Could you check a few things on this model? Use its own coordinates, in mm. Face numbers are marked on the shaded views. Round coordinates to 2 decimals unless told otherwise and drop trailing zeros. Loops run counter-clockwise (first coordinate to the right, second up) from the corner with the lowest first, then second, coordinate; pieces in that order, holes last.
from build123d import *

# Parameters (mm, degrees)
SKETCH097_W     = 172
SKETCH097_H     = 95
PAD059_DEPTH    = 4.5
SKETCH098_W     = 6
SKETCH098_H     = 19
POCKET036_DEPTH = 3
SKETCH099_W     = 6.3
SKETCH099_H     = 11
SKETCH099_W_2   = 6
POCKET037_DEPTH = 5
PAD060_DEPTH    = 16
POCKET038_DEPTH = 5
POCKET039_DEPTH = 9
SKETCH103_R     = 1.15
POCKET040_DEPTH = 5
SKETCH104_R     = 3.3
POCKET041_DEPTH = 3


with BuildPart() as part:
    # Sketch097 → Pad059 (new body)
    with BuildSketch(Plane.XZ):
        Rectangle(SKETCH097_W, SKETCH097_H)
    extrude(amount=PAD059_DEPTH)

    # Sketch098 (on Face6 of Pad059) → Pocket036 (cut)
    with BuildSketch(Plane.XZ.offset(4.5)):
        Polygon((64.5, 3), (69.5, 3), (69.5, 28.5), (75.5, 28.5), (75.5, 47.5), (56.5, 47.5), (56.5, 37.5), (64.5, 37.5), align=None)
        with Locations((39, 38)):
            Rectangle(SKETCH098_W, SKETCH098_H)
        Polygon((-64.5, 3), (-69.5, 3), (-69.5, 28.5), (-75.5, 28.5), (-75.5, 47.5), (-56.5, 47.5), (-56.5, 37.5), (-64.5, 37.5), align=None)
    extrude(amount=-POCKET036_DEPTH, mode=Mode.SUBTRACT)

    # Sketch099 (on Face26 of Pocket036) → Pocket037 (cut)
    with BuildSketch(Plane.XZ.offset(1.5)):
        with Locations((72.35, 42)):
            Rectangle(SKETCH099_W, SKETCH099_H)
        with Locations((39, 42)):
            Rectangle(SKETCH099_W_2, SKETCH099_H)
        with Locations((-72.35, 42)):
            Rectangle(SKETCH099_W, SKETCH099_H)
    extrude(amount=-POCKET037_DEPTH, mode=Mode.SUBTRACT)

    # Sketch100 (on Face5 of Pocket037) → Pad060 (join)
    with BuildSketch(Plane.XZ.offset(4.5)):
        Polygon((-69.5, 28.5), (-71.5, 28.5), (-71.5, 1), (-62.5, 1), (-62.5, 37.5), (-64.5, 37.5), (-64.5, 3), (-69.5, 3), align=None)
        Polygon((64.5, 37.5), (64.5, 3), (69.5, 3), (69.5, 28.5), (71.5, 28.5), (71.5, 1), (62.5, 1), (62.5, 37.5), align=None)
    extrude(amount=PAD060_DEPTH)

    # Sketch101 (on Face27 of Pad060) → Pocket038 (cut)
    with BuildSketch(Plane(origin=(-71.5, 0, 0), x_dir=(0, 0, -1), z_dir=(-1, 0, 0))):
        with BuildLine():
            ThreePointArc((-28.5, 4.5), (-18.161779, 10.994502), (-10.5, 20.5))
            Line((-28.5, 20.5), (-10.5, 20.5))
            Line((-28.5, 4.5), (-28.5, 20.5))
        make_face()
    extrude(amount=-POCKET038_DEPTH, mode=Mode.SUBTRACT)

    # Sketch102 (on Face22 of Pocket038) → Pocket039 (cut)
    with BuildSketch(Plane(origin=(62.5, 0, 0), x_dir=(0, 0, -1), z_dir=(-1, 0, 0))):
        with BuildLine():
            Line((-37.5, 20.5), (-10.5, 20.5))
            ThreePointArc((-28.5, 4.5), (-18.161779, 10.994501), (-10.5, 20.5))
            Line((-37.5, 4.5), (-28.5, 4.5))
            Line((-37.5, 20.5), (-37.5, 4.5))
        make_face()
    extrude(amount=-POCKET039_DEPTH, mode=Mode.SUBTRACT)

    # Sketch103 (on Face4 of Pocket039) → Pocket040 (cut)
    with BuildSketch(Plane(origin=(0, 0, 0), x_dir=(1, 0, 0), z_dir=(0, 1, 0))):
        with Locations((-83, 43.5)):
            Circle(SKETCH103_R)
        with Locations((83, 43.5)):
            Circle(SKETCH103_R)
        with Locations((83, -43.5)):
            Circle(SKETCH103_R)
        with Locations((-83, -43.5)):
            Circle(SKETCH103_R)
    extrude(amount=-POCKET040_DEPTH, mode=Mode.SUBTRACT)

    # Sketch104 (on Face4 of Pocket040) → Pocket041 (cut)
    with BuildSketch(Plane(origin=(0, 0, 0), x_dir=(1, 0, 0), z_dir=(0, 1, 0))):
        with Locations((83, 43.5)):
            Circle(SKETCH104_R)
        with Locations((83, -43.5)):
            Circle(SKETCH104_R)
        with Locations((-83, -43.5)):
            Circle(SKETCH104_R)
        with Locations((-83, 43.5)):
            Circle(SKETCH104_R)
    extrude(amount=-POCKET041_DEPTH, mode=Mode.SUBTRACT)


with BuildPart() as part_1:
    # Body021 placement: moved
    add(part.part.moved(Location((0, -4, -56))))


solid = part_1.part
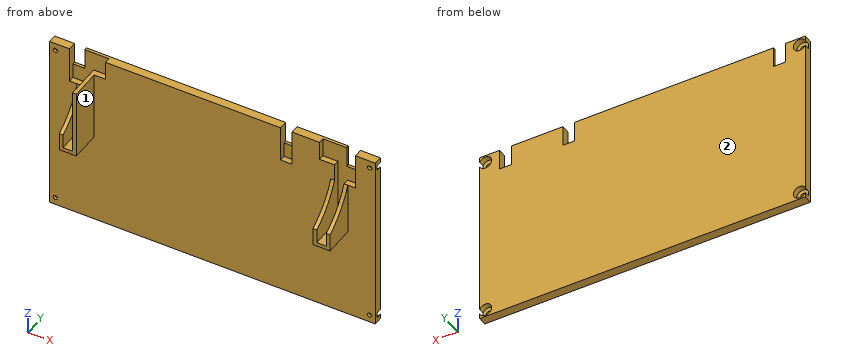
Item 1: If we section it at A-A, the plane y = -16.5: Please give me the cut outline in (x, z).
Results list:
outline: (-71.5, -55) - (-62.5, -55) - (-62.5, -18.5) - (-64.5, -18.5) - (-64.5, -53) - (-69.5, -53) - (-69.5, -39.43) - (-71.5, -39.43) - close; (62.5, -55) - (71.5, -55) - (71.5, -39.43) - (69.5, -39.43) - (69.5, -53) - (64.5, -53) - (64.5, -39.43) - (62.5, -39.43) - close
Item 2: If I drill on line 1 along X through (y, z) = (-19.75, -48); line 2 along Z through (x, y) = (-83, -7.5); line 3 along X through (y, z) = (-5.7, -12.5), over which ranges is the centre line in solid material (lowest first)?
Results list:
line 1: x = -71.5 to -69.5, -64.5 to -62.5, 62.5 to 64.5, 69.5 to 71.5
line 2: z = -103.5 to -100.65, -98.35 to -13.65, -11.35 to -8.5
line 3: x = -79.7 to -75.5, -56.5 to 36, 42 to 56.5, 75.5 to 79.7
Item 3: We'd pull the mould along X, two halves only. Please class the marked faces 1 and 2: released by +X, released by -X, zero draft, split by the parting line, or undercut.
Results list:
face 1: undercut
face 2: zero draft
Item 4: If we section it at B-B, the plane z = -50: Please give me the cut outline in (x, y).
Results list:
outline: (-86, -8.5) - (-71.5, -8.5) - (-71.5, -24.5) - (-69.5, -24.5) - (-69.5, -5.5) - (-64.5, -5.5) - (-64.5, -24.5) - (-62.5, -24.5) - (-62.5, -8.5) - (62.5, -8.5) - (62.5, -24.5) - (64.5, -24.5) - (64.5, -5.5) - (69.5, -5.5) - (69.5, -24.5) - (71.5, -24.5) - (71.5, -8.5) - (86, -8.5) - (86, -4) - (-86, -4) - close
Item 5: Will these pins go through, and if not, where does the flat tip stop? pin 1 (2.5 mm diameter, centred on x = 67, y = -11, fed in from +Z); pin 2 (5.5 mm diameter, centred on y = -13, z = -46, fed in from +X); pin 3 (4 mm diameter, centred on x = -62.5, y = -18, fed in from +Z).
Results list:
pin 1: stops at z = -53
pin 2: stops at x = 71.5
pin 3: stops at z = -18.5
Item 6: If we section it at C-C, the plane x = 40: Please give me the cut outline in (y, z).
Results list:
outline: (-8.5, -103.5) - (-4, -103.5) - (-4, -19.5) - (-5.5, -19.5) - (-5.5, -27.5) - (-8.5, -27.5) - close
Item 7: If we section it at D-D, the plane z = -29.5: Please give me the cut outline in (x, y).
Results list:
outline: (-86, -8.5) - (-71.5, -8.5) - (-71.5, -9.4) - (-69.5, -9.4) - (-69.5, -5.5) - (-64.5, -5.5) - (-64.5, -24.5) - (-62.5, -24.5) - (-62.5, -8.5) - (62.5, -8.5) - (62.5, -9.4) - (64.5, -9.4) - (64.5, -5.5) - (69.5, -5.5) - (69.5, -9.4) - (71.5, -9.4) - (71.5, -8.5) - (86, -8.5) - (86, -4) - (-86, -4) - close
